Autodesk Inventor part; units mm, degrees
ref_plane "YZ Plane" through (0, 0, 0) normal (1, 0, 0) x (0, 1, 0)
ref_plane "XZ Plane" through (0, 0, 0) normal (0, 1, 0) x (-1, 0, 0)
ref_plane "XY Plane" through (0, 0, 0) normal (0, 0, 1) x (1, 0, 0)
sketch "Sketch1" plane through (0, 0, 0) normal (0, 1, 0) x (-1, 0, 0)
  circle A0 centre (0, 0) radius 8.5
  dimension "d0" = 17
extrude "Extrusion1" add sketch "Sketch1" along normal blind 124
sketch "Sketch2" plane through (0, 124, 0) normal (0, 1, 0) x (1, 0, 0)
  line L0 (6, 6) -> (-6, 6)
  line L1 (-6, 6) -> (-6, -6)
  line L2 (-6, -6) -> (6, -6)
  line L3 (6, -6) -> (6, 6)
  line L4 (6, 6) -> (-6, -6) construction
  line L5 (-6, 6) -> (6, -6) construction
  point P0 (0, 0)
  dimension "d3" = 12
  dimension "d4" = 12
extrude "Extrusion2" add sketch "Sketch2" along normal blind 18
sketch "Sketch3" plane through (0, 142, 0) normal (0, 1, 0) x (1, 0, 0)
  circle A0 centre (0, 0) radius 6
  line L0 (-6, 6) -> (-6, -6)
  line L1 (6, 6) -> (-6, 6)
  line L2 (6, -6) -> (6, 6)
  line L3 (-6, -6) -> (6, -6)
extrude "Extrusion3" add sketch "Sketch3" along normal blind 16 contours A0
sketch "Sketch4" plane through (0, 0, 0) normal (0, -1, 0) x (1, 0, 0)
  circle A0 centre (0, 0) radius 8.5
  circle A1 centre (0, 0) radius 10
  dimension "d9" = 20
extrude "Extrusion4" add sketch "Sketch4" along normal blind 28 contours A0 | A1
sketch "Sketch5" plane through (0, -28, 0) normal (0, -1, 0) x (1, 0, 0)
  circle A0 centre (0, 0) radius 8.5
  dimension "d12" = 17
extrude "Extrusion5" add sketch "Sketch5" along normal blind 23
chamfer "Chamfer1" distance 1.5 angle 45 2 edges at (-10, -28, 0) (-10, 0, 0)
sketch "Sketch6" plane through (0, 0, 0) normal (0, 0, 1) x (1, 0, 0)
  line L0 (-8.5, -51) -> (8.5, -51)
  arc A0 (0, -53.2776) -> (8.5, -51) centre (0, -36.2776) ccw
  line L1 (0, -51) -> (0, -53.2776)
  point P0 (0, 0)
revolve "Revolution1" add sketch "Sketch6" angle 360 about axis through (0, -51, 0) along (0, -1, 0)
thread "Thread1"
thread "Thread2"
properties part number "00.32.010 \"Spindle\"" material "Steel"
Can you work these out from the model? Positions are in its coordinate system, mm. A direction names the side the tool comes from. Give positions to 0.01 mm unless a question says otherwise; leave off trailing zeros. Order: outer loops, then holes, each group sorted by start corner. A loop starts at its lowest first (then second) coordinate and runs counter-clockwise, first axis right, second up. Notation, with made-up numbers: (-26.5, 35) - (23.5, 35) arc R32 cw to (23.5, 70) - close; hole circle Ø5 at (36, 8). An arc over 180 degrees is marked (long way). Use a Markdown table: item, result. Add a question column.
Q1. If we section it at A-A on y = -13: Write out the boundary of the cut face in (x, z), plus the area to 3 significant figures.
Q2. I'm going to push flat-ended pins straight in: pin 1 (9.5 mm diameter, centred on x = 3, y = 135, fed in from +Z); pin 2 (3.5 mm diameter, centred on x = -2, y = 129, fed in from -Z); pin 3 (4 mm diameter, centred on x = -7.5, z = -6.5, fed in from +Y). Where does each tip first touch, or does it pass through?
Q3. If we section it at B-B on y = 114.5: Write out the boundary of the cut face in (x, z), plus the area to 3 significant figures.
Q4. Please list where these lines run through material, in increasing order: line 1 along Y through (x, z) = (0.5, -1); line 2 along Z through (x, y) = (-2.5, 137); line 3 along X through (y, z) = (34, 1.25).
Q5. On a 3-axis mill with a long thin cutter (end or side, diameter ignored), from which of +Z, -Z, +X, -X, +Y, -Y can I reach the whole of each face in a straight line? I mean faces 1 (the flat face through (5, 142, 5)), 2 (the flat face through (0, 133, -6)), 3 (the flat face through (-6, 133, 0)), 4 (the flat face through (-0.6, 124, -6.3)). Say none if no direction works.
Answers follow:
| question | item | result |
|---|---|---|
| 1 | outline | circle Ø20 at (0, 0) |
| 1 | area | 314 mm^2 |
| 2 | pin 1 | stops at z = 6 |
| 2 | pin 2 | stops at z = -6 |
| 2 | pin 3 | stops at y = 142 |
| 3 | outline | circle Ø17 at (0, 0) |
| 3 | area | 227 mm^2 |
| 4 | line 1 | y = -53.24 to 158 |
| 4 | line 2 | z = -6 to 6 |
| 4 | line 3 | x = -8.41 to 8.41 |
| 5 | face 1 | +Z, +X, +Y |
| 5 | face 2 | -Z, +X, -X, +Y |
| 5 | face 3 | +Z, -Z, -X, +Y |
| 5 | face 4 | +Y |
